Geometry: final body of the model. Coordinates: model frame, mm. Give positions to 0.01 mm unless a question says otherwise; leave off trailing zeros. Write each loop counter-clockwise with the first axis right and the second up, starting at its lowest first coordinate (ties: lowest second). Pieces come first, ordered by that corner, then holes. Notation, with made-up numbers: (83.5, 24) -> (88.5, 24) arc R23 cw to (88.5, 43) -> close; hole circle Ø3 at (31.25, 63). An arc over 180 degrees is marked (long way). Answer as a JSON object with one key per item and string values. Group by question number.
(1) Section query C-C on x = 0. State how many separate pieces and enclosed holes the cut face has, plus the area to 4 significant figures.
(2) Contact query for flat-ended pins moving along their axis: pin 1 Ø2 at (x, y) = (0, 8) entering from -Z; pin 2 Ø4 at (x, z) = (7.5, 2) entering from +Y; pin 3 Ø2 at (y, z) = (-4, 0.5) entering from -X. Output: stop coordinate, or through.
(3) Section query A-A on y = 0. Output: boundary loops of the cut face in (x, z).
(4) Material intervals for probe 1 along Z at (x, y) = (9, 3.5); probe 2 along Y at (x, z) = (0, 3.35); probe 3 along Y at (x, z) = (-7.5, 3.25), sorted ascending.
(5) Draft query along X for faces 1 (the face through (10, 3.2, 3.3)), 2 (the face through (-6.35, -5.11, 3.26)), 3 (the face through (2.1, 2.4, 4)). Return one class per face: +X half, -X half, draft (parallel to the pull), parting line (faces both ways), or undercut.
(6) Section query B-B on z = 0.75. Output: boundary loops of the cut face in (x, y).
from build123d import *

# Parameters (mm, degrees)
SKETCH1_R                = 10.5
BOSS_EXTRUDE1_DEPTH      = 4
BOSS_EXTRUDE1_DEPTH_BACK = 4
SKETCH2_R                = 3
CUT_EXTRUDE1_DEPTH       = 10
CHAMFER1_SIZE            = 0.25
CHAMFER2_SIZE            = 0.25
CUT_EXTRUDE2_START       = -1.5
SKETCH3_OUTSIDE_W        = 29.152
SKETCH3_OUTSIDE_H        = 29.152
SKETCH3_OUTSIDE_R        = 5
CUT_EXTRUDE2_DEPTH       = 5
CHAMFER3_SIZE            = 0.25
SKETCH4_R                = 1.25
CUT_EXTRUDE3_DEPTH       = 1
CUT_EXTRUDE3_DEPTH_BACK  = 9


with BuildPart() as part:
    # Sketch1 → Boss-Extrude1 (new body, two sides)
    with BuildSketch(Plane.XY) as boss_extrude1_sk:
        Circle(SKETCH1_R)
    extrude(amount=BOSS_EXTRUDE1_DEPTH)
    extrude(boss_extrude1_sk.sketch, amount=-BOSS_EXTRUDE1_DEPTH_BACK)

    # Sketch2 → Cut-Extrude1 (cut)
    with BuildSketch(Plane.XY.offset(4)):
        Circle(SKETCH2_R)
    extrude(amount=-CUT_EXTRUDE1_DEPTH, mode=Mode.SUBTRACT)

    # Chamfer1
    chamfer1_edges = [part.edges().sort_by_distance(p)[0] for p in [
        (-10.5, 0, 4),
    ]]
    chamfer(chamfer1_edges, length=CHAMFER1_SIZE)

    # Chamfer2
    chamfer2_edges = [part.edges().sort_by_distance(p)[0] for p in [
        (-10.5, 0, -4),
    ]]
    chamfer(chamfer2_edges, length=CHAMFER2_SIZE)

    # Sketch3 outside → Cut-Extrude2 (cut)
    with BuildSketch(Plane.XY.offset(4).offset(CUT_EXTRUDE2_START)):
        Rectangle(SKETCH3_OUTSIDE_W, SKETCH3_OUTSIDE_H)
        Circle(SKETCH3_OUTSIDE_R, mode=Mode.SUBTRACT)
    extrude(amount=-CUT_EXTRUDE2_DEPTH, mode=Mode.SUBTRACT)

    # Chamfer3
    chamfer3_edges = [part.edges().sort_by_distance(p)[0] for p in [
        (-10.5, 0, 2.5),
        (-10.5, 0, -2.5),
    ]]
    chamfer(chamfer3_edges, length=CHAMFER3_SIZE)

    # Sketch4 → Cut-Extrude3 (cut, two sides)
    with BuildSketch(Plane.XY.offset(4)) as cut_extrude3_sk:
        with Locations((0, 8)):
            Circle(SKETCH4_R)
        with Locations((6.92820323, 4)):
            Circle(SKETCH4_R)
        with Locations((6.92820323, -4)):
            Circle(SKETCH4_R)
        with Locations((0, -8)):
            Circle(SKETCH4_R)
        with Locations((-6.92820323, -4)):
            Circle(SKETCH4_R)
        with Locations((-6.92820323, 4)):
            Circle(SKETCH4_R)
    extrude(amount=CUT_EXTRUDE3_DEPTH, mode=Mode.SUBTRACT)
    extrude(cut_extrude3_sk.sketch, amount=-CUT_EXTRUDE3_DEPTH_BACK, mode=Mode.SUBTRACT)


solid = part.part
Answer list:
{
 "1": {"separate pieces": "6", "enclosed holes": "0", "area": "49.75 mm2"},
 "2": {"pin 1": "through", "pin 2": "y = 8.85", "pin 3": "x = -4"},
 "3": {"outline": "(-10.5, -3.75) -> (-10.25, -4) -> (-3, -4) -> (-3, 4) -> (-10.25, 4) -> (-10.5, 3.75) -> (-10.5, 2.75) -> (-10.25, 2.5) -> (-5, 2.5) -> (-5, -2.5) -> (-10.25, -2.5) -> (-10.5, -2.75) -> close; (3, -4) -> (10.25, -4) -> (10.5, -3.75) -> (10.5, -2.75) -> (10.25, -2.5) -> (5, -2.5) -> (5, 2.5) -> (10.25, 2.5) -> (10.5, 2.75) -> (10.5, 3.75) -> (10.25, 4) -> (3, 4) -> close"},
 "4": {"probe 1": "-4 to -2.5, 2.5 to 4", "probe 2": "-10.5 to -9.25, -6.75 to -3, 3 to 6.75, 9.25 to 10.5", "probe 3": "-7.35 to -5.11, -2.89 to 2.89, 5.11 to 7.35"},
 "5": {"face 1": "parting line", "face 2": "undercut", "face 3": "draft"},
 "6": {"outline": "circle Ø10 at (0, 0); hole circle Ø6 at (0, 0)"}
}
